Geometry check sheet. Reference: the model listing, model coordinates, mm. A direction names the side the tool comes from. Round coordinates to 2 decimals unless told otherwise and drop trailing zeros. Loops run counter-clockwise (first coordinate to the right, second up) from the corner with the lowest first, then second, coordinate; pieces in that order, holes last. Notation, with made-up numbers: (43.5, 51) -> (87.5, 51) arc R15 cw to (87.5, 79) -> close; hole circle Ø4 at (-27.75, -22.5). An arc over 180 degrees is marked (long way). Use a Markdown table: item, result. Add a question column.
Q1. Sectioned sample at C-C, the plane y = 107.5. Enter the section's corners in (x, z).
Q2. Sectioned sample at B-B, the plane x = 15. Enter the section's corners in (y, z).
Q3. Set-up check for faces 5 (the face through (15, 35, 110)), 6 (the face through (15, 30, -120)), 7 (the face through (30, 9, 11)): record each of +Z, -Z, +X, -X, +Y, -Y from which the full face is reachable in a straight line by a thin tool's end or side.
Q4. Gauge pin test, flat ends, axial feed: P1, Ø4, axis at x = 25.5, y = 74, coming from the -Z side; P2, Ø15, axis at x = 15, y = 42, coming from the +Z side; P3, Ø3, axis at x = 19, y = 134.5, coming from the -Z side. Record the tip position at first contact, or that the pin passes through.
Q5. Sectioned sample at D-D, the plane y = 26. Enter the section's corners in (x, z).
Q6. Release check for a two-part mould opening along Y. For faces 1 (the face through (8, 0, -2)), 2 (the face through (15, 30, 120)), 3 (the face through (15, 35, -110)), 4 (the face through (8, 10, 2)) record: released by +Y, released by -Y, zero draft, split by the parting line, or undercut.
Q7. Sectioned sample at A-A, the plane z = -115. Enter the section's corners in (x, y), then the cut area to 3 significant figures.
Q8. Material ranges on L1, parallel to Z at x = 15.5, y = 107.5; L2, parallel to Z at x = 15, y = 6.5; L3, parallel to X at y = 6, z = 0, recorded low to high.
```python
from build123d import *

# Parameters (mm, degrees)
EXTRUDE_THIN2_DEPTH     = 30
SKETCH2_R               = 47.5
SKETCH2_R_2             = 37.5
EXTRUDE_THIN3_DEPTH     = 30
SKETCH3_R               = 6
CUT_EXTRUDE1_DEPTH      = 146
CUT_EXTRUDE1_DEPTH_BACK = 11


with BuildPart() as part:
    # Sketch1 → Extrude-Thin2 (new body)
    with BuildSketch(Plane(origin=(0, 0, 0), x_dir=(0, 0, -1), z_dir=(1, 0, 0))):
        Polygon((0, 0), (120, 0), (120, 70), (110, 70), (110, 10), (0, 10), align=None)
    extrude(amount=EXTRUDE_THIN2_DEPTH)

    # Sketch2 → Extrude-Thin3 (add)
    with BuildSketch(Plane(origin=(30, 0, 0), x_dir=(0, 0, -1), z_dir=(1, 0, 0))):
        with Locations((115, 107.5)):
            Circle(SKETCH2_R)
        with Locations((115, 107.5)):
            Circle(SKETCH2_R_2, mode=Mode.SUBTRACT)
    extrude(amount=-EXTRUDE_THIN3_DEPTH)

    # Mirror1: part across plane


with BuildPart() as part_1:
    add(part.part)
    add(part.part.mirror(Plane(origin=(30, 0, 0), x_dir=(1, 0, 0), z_dir=(0, 0, 1))))

    # Sketch3 → Cut-Extrude1 (cut, two sides)
    with BuildSketch(Plane(origin=(0, 10, 0), x_dir=(1, 0, 0), z_dir=(0, 1, 0))) as cut_extrude1_sk:
        with Locations((15, 0)):
            Circle(SKETCH3_R)
    extrude(amount=CUT_EXTRUDE1_DEPTH, mode=Mode.SUBTRACT)
    extrude(cut_extrude1_sk.sketch, amount=-CUT_EXTRUDE1_DEPTH_BACK, mode=Mode.SUBTRACT)


solid = part_1.part
```
Values:
| question | item | result |
|---|---|---|
| 1 | outline | (0, -162.5) -> (30, -162.5) -> (30, -152.5) -> (0, -152.5) -> close; (0, -77.5) -> (30, -77.5) -> (30, -67.5) -> (0, -67.5) -> close; (0, 67.5) -> (30, 67.5) -> (30, 77.5) -> (0, 77.5) -> close; (0, 152.5) -> (30, 152.5) -> (30, 162.5) -> (0, 162.5) -> close |
| 2 | outline | (0, -120) -> (60.26, -120) arc R47.5 ccw (long way) to (60.26, -110) -> (10, -110) -> (10, -6) -> (0, -6) -> close; (0, 6) -> (10, 6) -> (10, 110) -> (60.26, 110) arc R47.5 ccw (long way) to (60.26, 120) -> (0, 120) -> close; hole circle Ø75 at (107.5, -115); hole circle Ø75 at (107.5, 115) |
| 3 | face 5 | +X, -X |
| 3 | face 6 | -Z, +X, -X, -Y |
| 3 | face 7 | +Z, -Z, +X, +Y, -Y |
| 4 | P1 | z = -150.55 |
| 4 | P2 | z = 120 |
| 4 | P3 | z = -155.07 |
| 5 | outline | (0, -120) -> (30, -120) -> (30, -110) -> (0, -110) -> close; (0, 110) -> (30, 110) -> (30, 120) -> (0, 120) -> close |
| 6 | face 1 | released by -Y |
| 6 | face 2 | zero draft |
| 6 | face 3 | undercut |
| 6 | face 4 | undercut |
| 7 | outline | (0, 0) -> (30, 0) -> (30, 70) -> (0, 70) -> close; (0, 145) -> (30, 145) -> (30, 155) -> (0, 155) -> close |
| 7 | area | 2,400 mm^2 |
| 8 | L1 | -162.5 to -152.5, -77.5 to -67.5, 67.5 to 77.5, 152.5 to 162.5 |
| 8 | L2 | -120 to -6, 6 to 120 |
| 8 | L3 | 0 to 9, 21 to 30 |
